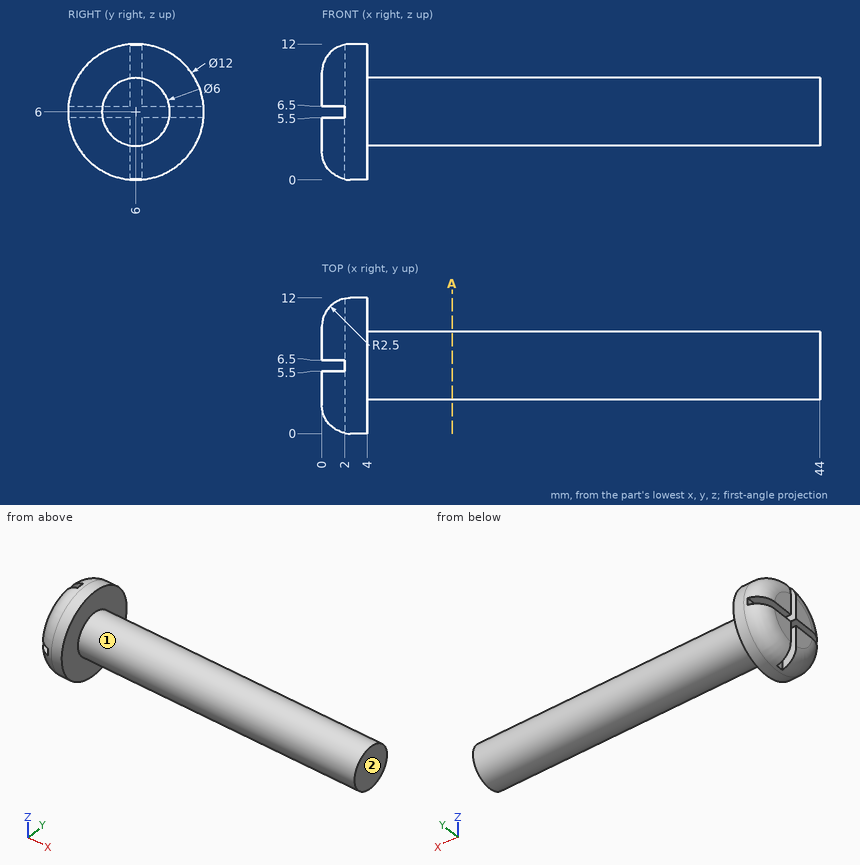
The figure shows three views and two pictorial views of one solid part (mm, origin at its lowest corner). Answer the questions. A direction names the side the tool comes from. Give positions to 0.01 mm unless a question says otherwise; leave off trailing zeros. Write each loop counter-clockwise with the first axis right and the second up, starting at its lowest first coordinate (ties: lowest second). Pieces come first, ordered by that corner, then holes.
Q1. Given pin 1 (2 mm diameter, centred on x = 32, z = 1.5, fed in from +Y); pin 2 (1 mm diameter, centred on x = 1, z = 2, fed in from -Y); pin 3 (2 mm diameter, centred on x = 11, y = 5, fed in from +Z); pin 4 (2 mm diameter, centred on x = 1, z = 10, fed in from +Y), each flat-ended and moving along its own axis, determine where each tip first touches the part or whether it passes through.
Answer:
pin 1: passes through
pin 2: stops at y = 1.59
pin 3: stops at z = 9
pin 4: stops at y = 10.88
Q2. A tool of negligible diameter and unlimited length cuts with its end or side. For the marked faces 1 and 2, from which of +Z, -Z, +X, -X, +Y, -Y can it reach the whole face along a straight path? Write none if from no direction.
Answer:
face 1: +X
face 2: +Z, -Z, +X, +Y, -Y
Q3. The part is cut by section A-A on x = 11.5. Give the vertices of the cut face in (y, z).
Answer:
outline: circle Ø6 at (6, 6)
Q4. Straight lines are drawn through the part: L1, parallel to Y at x = 41.5, z = 6; L2, parallel to X at y = 9.75, z = 7.25; L3, parallel to X at y = 1.25, z = 7.75. For each, find the intervals that lie inside material, in ascending order.
Answer:
L1: y = 3 to 9
L2: x = 0.04 to 4
L3: x = 0.55 to 4
